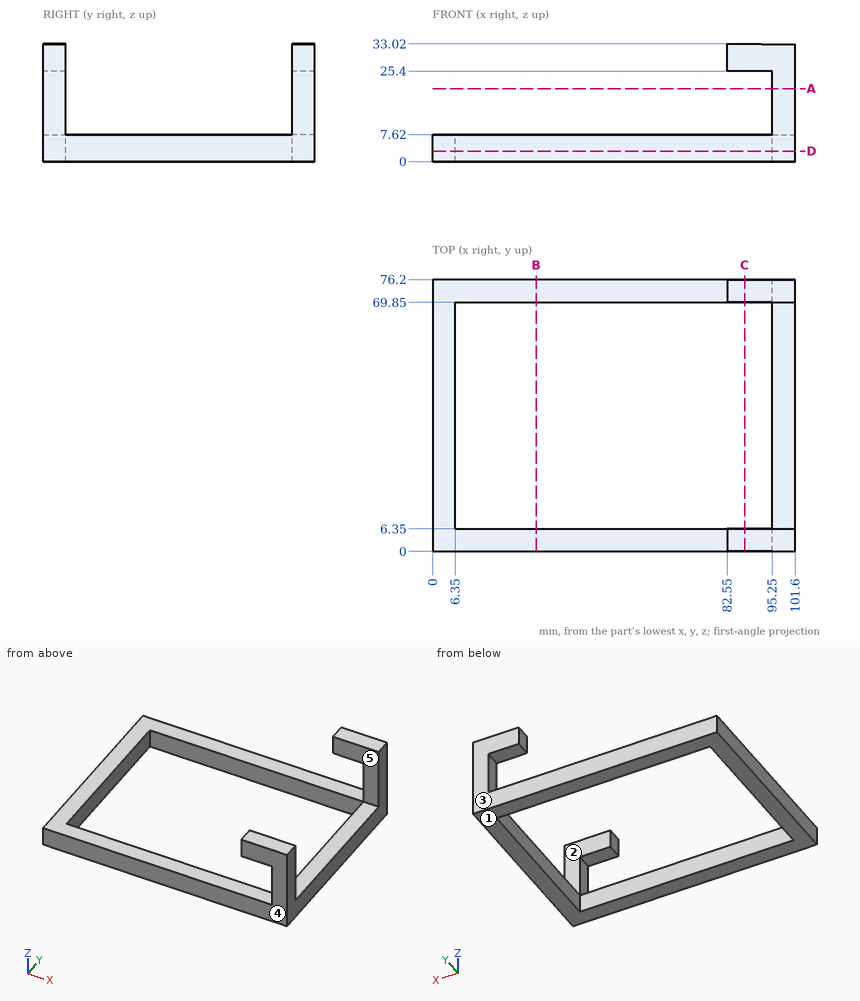
The figure shows three views and two pictorial views of one solid part (mm, origin at its lowest corner). Answer the questions. A direction names the side the tool comes from. Round coordinates to 2 decimals unless told otherwise and drop trailing zeros. Loops run counter-clockwise (first coordinate to the right, second up) from the corner with the lowest first, then second, coordinate; pieces in that order, holes last. Notation, with made-up numbers: (12, 60.5) - (49, 60.5) arc R20 cw to (49, 83.5) - close; hole circle Ø9 at (77, 19). An arc over 180 degrees is marked (long way). Use one line per item in the form item = value. Start each with the question number.
(1) Determine the mould class of the marked faces 3, 4 and 5 for opening direction Y: +Y half, -Y half, draft (parallel to the pull), parting line (faces both ways), or undercut.
(2) Find section B-B on x = 29. Determine the outline of the cut face in (y, z).
(3) Flat-ended cylindrical pins translate along their axes: P1, Ø12, axis at y = 59.5, z = 15, coming from the +X side; P2, Ø1.9, axis at y = 3.5, z = 18, coming from the -X side; P3, Ø1.9, axis at y = 4, z = 31, coming from the -X side; P4, Ø1.9, axis at x = 97, y = 32, coming from the +Z side. Find the tip coordinate at first contact, or state that the pin passes through.
(4) Which of the six approach directions +Z, -Z, +X, -X, +Y, -Y give full straight-line access (tool end or side, diameter ignored) to the marked faces 1 and 2?
(5) Find section D-D on z = 3. Determine the outline of the cut face in (x, y).
(6) Find section C-C on x = 87.5. Determine the outline of the cut face in (y, z), and give its area (3 significant figures).
(7) Consider line 1 (Y direction, x = 29, z = 2.5); line 2 (X direction, y = 9.5, z = 3.5); line 3 (Z direction, x = 5.5, y = 65). Determine where each line is inside the solid, lowest interval first.
(8) Find section A-A on z = 20.5. Determine the outline of the cut face in (x, y).
Answer list:
q1.face_3 = +Y half
q1.face_4 = -Y half
q1.face_5 = undercut
q2.outline = (0, 0) - (6.35, 0) - (6.35, 7.62) - (0, 7.62) - close; (69.85, 0) - (76.2, 0) - (76.2, 7.62) - (69.85, 7.62) - close
q3.P1 = through
q3.P2 = 95.25
q3.P3 = 82.55
q3.P4 = 7.62
q4.face_1 = -Z, +X, -X, +Y, -Y
q4.face_2 = +Z, +X, -X
q5.outline = (0, 0) - (101.6, 0) - (101.6, 76.2) - (0, 76.2) - close; hole (6.35, 6.35) - (95.25, 6.35) - (95.25, 69.85) - (6.35, 69.85) - close
q6.outline = (0, 0) - (6.35, 0) - (6.35, 7.62) - (0, 7.62) - close; (0, 25.4) - (6.35, 25.4) - (6.35, 33.02) - (0, 33.02) - close; (69.85, 0) - (76.2, 0) - (76.2, 7.62) - (69.85, 7.62) - close; (69.85, 25.4) - (76.2, 25.4) - (76.2, 33.02) - (69.85, 33.02) - close
q6.area = 194 mm^2
q7.line_1 = 0 to 6.35, 69.85 to 76.2
q7.line_2 = 0 to 6.35, 95.25 to 101.6
q7.line_3 = 0 to 7.62
q8.outline = (95.25, 0) - (101.6, 0) - (101.6, 6.35) - (95.25, 6.35) - close; (95.25, 69.85) - (101.6, 69.85) - (101.6, 76.2) - (95.25, 76.2) - close
